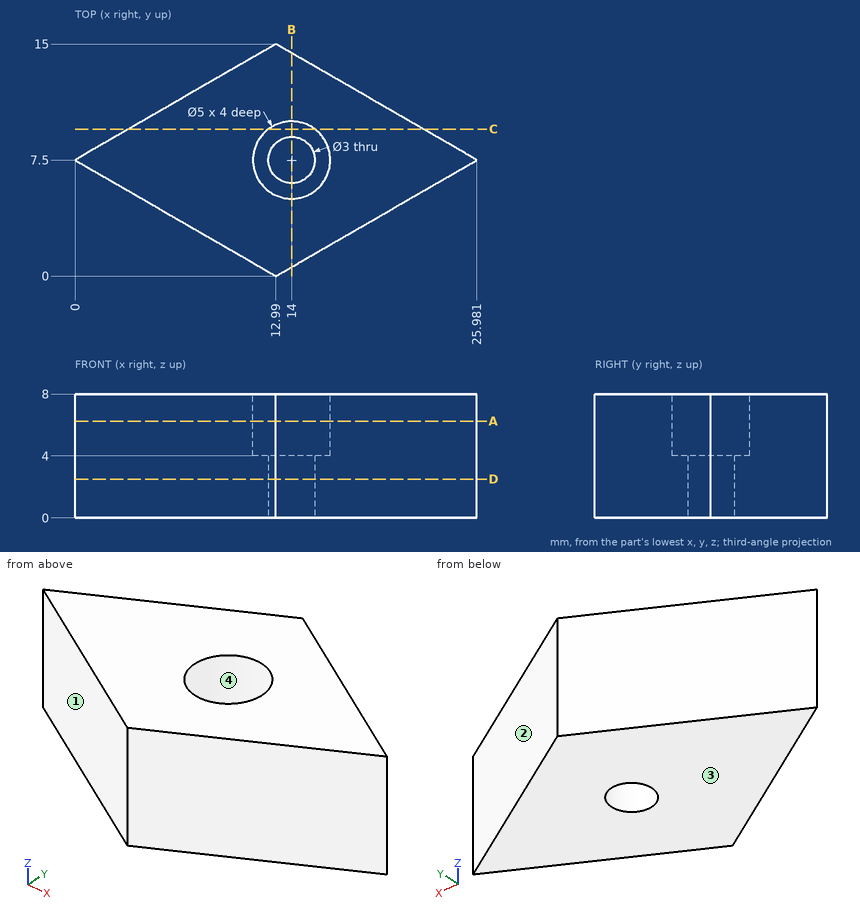
Geometry: see drawing. Coordinates: mm, zero at the bounding-box minimum. Round coordinates to 2 decimals unless told otherwise and drop trailing zeros. Write each loop counter-clockwise with the first axis right and the second up, starting at its lowest first coordinate (ties: lowest second). Pieces come first, ordered by that corner, then holes. Notation, with made-up numbers: M 84,-8 L 112,-8 A30 ccw 112,20 Z; hole C 85,-40 d2. An arc over 180 degrees is marked long. Answer in a Markdown table with one row per item. Add a question column.
(1) Cut plane C-C, the plane y = 9.5. Return the cut outline in (x, z), then the cut area to 3 significant figures.
(2) Cut plane A-A, the plane z = 6.25. Return the cut outline in (x, y).
(3) Draft query along Y for the marked faces 1, 2, 3 and 4. Return one class per face: pulls with the +Y half, pulls with the -Y half, needs draft (parallel to the pull), parting line crosses it, or undercut.
(4) Cut plane B-B, the plane x = 14. Return the cut outline in (y, z).
(5) Ray query, L1, parallel to Y at x = 14, z = 7.25; L2, parallel to Y at x = 12.5, z = 5.25 (1 decimal); L3, parallel to Z at x = 16, y = 7.5. Return the intervals inside material, ascending.
(6) Cut plane D-D, the plane z = 2.5. Return the cut outline in (x, y), then the cut area to 3 significant figures.
(7) Contact query for flat-ended pins moving along their axis: pin 1 (2 mm diameter, centred on x = 9.5, z = 5.5, fed in from -Y); pin 2 (4 mm diameter, centred on x = 7.5, z = 5, fed in from -Y) (1 decimal); pin 3 (4 mm diameter, centred on y = 5, z = 3, fed in from +X) (1 decimal). Output: stop coordinate, or through.
Established:
| question | item | result |
|---|---|---|
| 1 | outline | M 3.46,0 L 22.52,0 L 22.52,8 L 15.5,8 L 15.5,4 L 12.5,4 L 12.5,8 L 3.46,8 Z |
| 1 | area | 140 mm² |
| 2 | outline | M 0,7.5 L 12.99,0 L 25.98,7.5 L 12.99,15 Z; hole C 14,7.5 d5 |
| 3 | face 1 | pulls with the -Y half |
| 3 | face 2 | pulls with the +Y half |
| 3 | face 3 | needs draft |
| 3 | face 4 | undercut |
| 4 | outline | M 0.58,0 L 6,0 L 6,4 L 5,4 L 5,8 L 0.58,8 Z; M 9,0 L 14.42,0 L 14.42,8 L 10,8 L 10,4 L 9,4 Z |
| 5 | L1 | 0.58 to 5, 10 to 14.42 |
| 5 | L2 | 0.3 to 5.5, 9.5 to 14.7 |
| 5 | L3 | 0 to 4 |
| 6 | outline | M 0,7.5 L 12.99,0 L 25.98,7.5 L 12.99,15 Z; hole C 14,7.5 d3 |
| 6 | area | 188 mm² |
| 7 | pin 1 | y = 1.44 |
| 7 | pin 2 | y = 2 |
| 7 | pin 3 | x = 25.1 |
